Check sheet for the drawn part. Datum: minimum x, y, z corner. Units: mm. A direction names the side the tool comes from. Give positions to 0.01 mm unless a question says otherwise; leave off trailing zeros. Write each loop counter-clockwise with the first axis right and the second up, starting at its lowest first coordinate (ties: lowest second). Pieces come first, ordered by that corner, then holes. Notation, with made-up numbers: (-23.75, 70) - (-3.75, 70) arc R29 cw to (-3.75, 95) - close; hole circle Ø4 at (-23.75, 69.25). An arc over 180 degrees is marked (long way). Use a Markdown table: item, result.
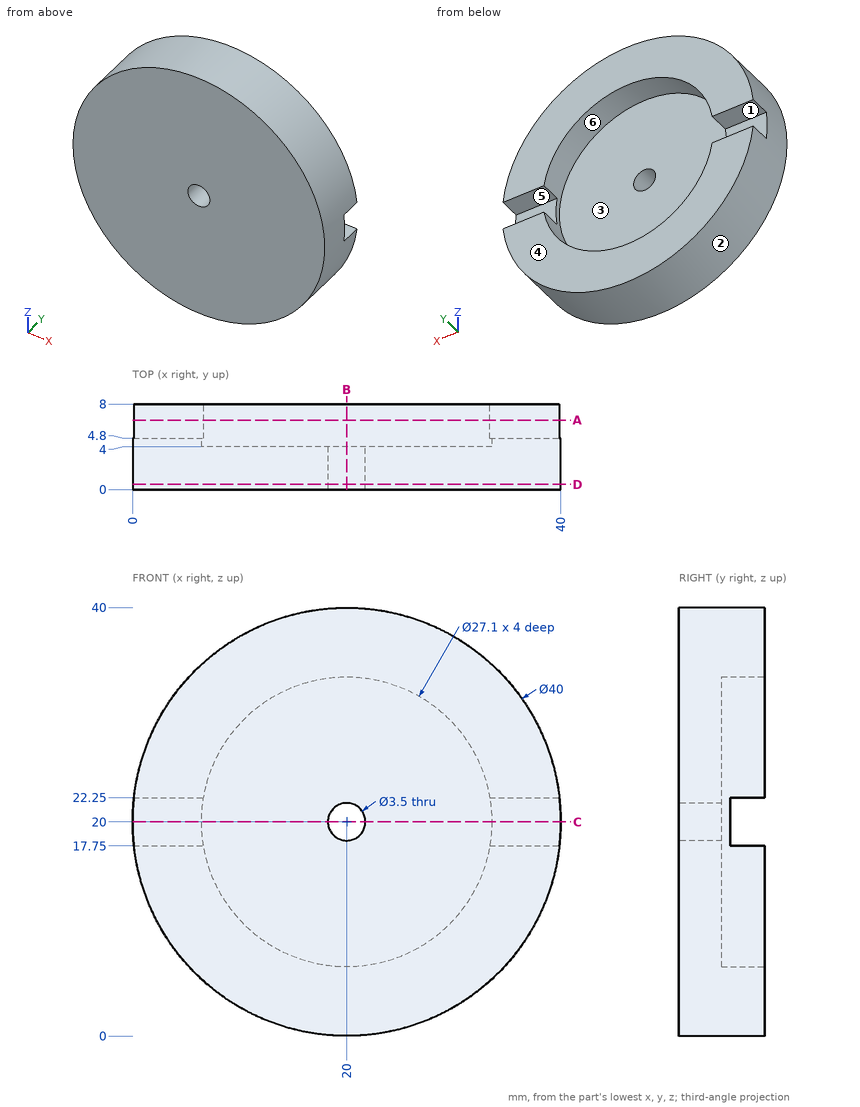
1) Depth check by flat-ended pin: P1, Ø2.5, axis at x = 3.5, z = 20, coming from the +Y side; P2, Ø3.5, axis at x = 37, y = 6.5, coming from the +Z side; P3, Ø3.5, axis at x = 3, y = 6.5, coming from the -Z side. Enter the tip coordinate at first touch or a pass-through.
Working result:
| item | result |
|---|---|
| P1 | stops at y = 4.8 |
| P2 | stops at z = 32.94 |
| P3 | stops at z = 7.06 |
2) Mould release check, pull along X, two halves, no side actions. Record for the marked faces 1, 2 and 3: pulls with the +X half, pulls with the -X half, needs draft (parallel to the pull), parting line crosses it, or undercut.
Working result:
| item | result |
|---|---|
| face 1 | needs draft |
| face 2 | parting line crosses it |
| face 3 | undercut |
3) Set-up check for the marked faces 4, 5 and 6: record each of +Z, -Z, +X, -X, +Y, -Y from which the full face is reachable in a straight line by a thin tool's end or side.
Working result:
| item | result |
|---|---|
| face 4 | +Z, -Z, +X, -X, +Y |
| face 5 | +X, -X, +Y |
| face 6 | +Y |
4) Material ranges on L1, parallel to Z at x = 20, y = 5.35; L2, parallel to Z at x = 20, y = 2.35; L3, parallel to Y at x = 20, z = 23.5, recorded low to high. Write a range as from..to.
Working result:
| item | result |
|---|---|
| L1 | z = 0..6.45, 33.55..40 |
| L2 | z = 0..18.25, 21.75..40 |
| L3 | y = 0..4 |
5) Section check A-A on y = 6.5. Record the boundary of the cut face in (x, z), then the cut area to 3 significant figures.
Working result:
| item | result |
|---|---|
| outline | (0.13, 17.75) arc R20 ccw to (39.87, 17.75) - (33.36, 17.75) arc R13.55 cw to (6.64, 17.75) - close; (0.13, 22.25) - (6.64, 22.25) arc R13.55 cw to (33.36, 22.25) - (39.87, 22.25) arc R20 ccw to start |
| area | 622 mm² |
6) Section check C-C on z = 20. Record the boundary of the cut face in (x, y), then the cut area to 3 significant figures.
Working result:
| item | result |
|---|---|
| outline | (0, 0) - (18.25, 0) - (18.25, 4) - (6.45, 4) - (6.45, 4.8) - (0, 4.8) - close; (21.75, 0) - (40, 0) - (40, 4.8) - (33.55, 4.8) - (33.55, 4) - (21.75, 4) - close |
| area | 156 mm² |
7) Section check B-B on x = 20. Record the boundary of the cut face in (y, z), then the cut area to 3 significant figures.
Working result:
| item | result |
|---|---|
| outline | (0, 0) - (8, 0) - (8, 6.45) - (4, 6.45) - (4, 18.25) - (0, 18.25) - close; (0, 21.75) - (4, 21.75) - (4, 33.55) - (8, 33.55) - (8, 40) - (0, 40) - close |
| area | 198 mm² |
8) Section check D-D on y = 0.5. Record the boundary of the cut face in (x, z).
Working result:
| item | result |
|---|---|
| outline | circle Ø40 at (20, 20); hole circle Ø3.5 at (20, 20) |
